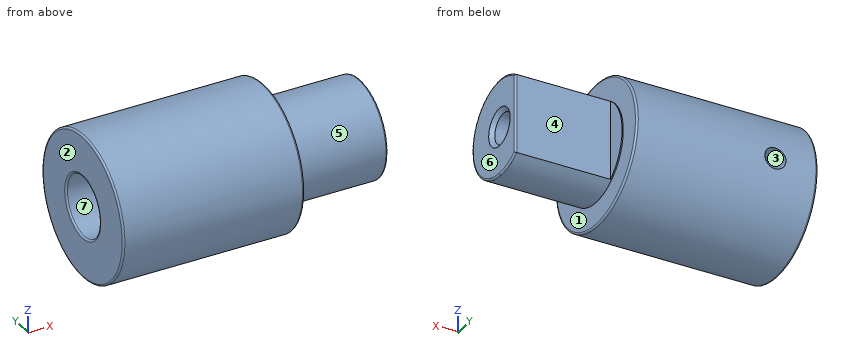
from build123d import *

# Parameters (mm, degrees)
CUT_EXTRUDE1_DEPTH          = 7.9
M3_TAPPED_HOLE1_D           = 2.5
M3_TAPPED_HOLE1_CSINK_D     = 3.15
M3_TAPPED_HOLE1_CSINK_ANGLE = 90
FILLET1_R                   = 0.15
SKETCH6_R                   = 0.875
CUT_EXTRUDE2_DEPTH          = 6


with BuildPart() as part:
    # Sketch2 → Revolve1 (revolve)
    with BuildSketch(Plane(origin=(0, 0, 0), x_dir=(1, 0, 0), z_dir=(0, 1, 0))):
        Polygon((0, 2.5), (13.1, 2.5), (13.1, 0), (23, 0), (23, 4), (15, 4), (15, 5.95), (0, 5.95), align=None)
    revolve(axis=Axis((0, 0, 0), (1, 0, 0)))

    # Sketch3 → Cut-Extrude1 (cut)
    with BuildSketch(Plane(origin=(23, 0, 0), x_dir=(0, 0, -1), z_dir=(1, 0, 0))):
        with BuildLine():
            Line((-3.272613634, 2.3), (3.272613634, 2.3))
            ThreePointArc((3.272613634, 2.3), (0, 4), (-3.272613634, 2.3))
        make_face()
    extrude(amount=-CUT_EXTRUDE1_DEPTH, mode=Mode.SUBTRACT)

    # M3 Tapped Hole1 (through all)
    with Locations(Plane(origin=(23, 0, 0), x_dir=(0, 0, 1), z_dir=(1, 0, 0))):
        with Locations((0, 0)):
            CounterSinkHole(M3_TAPPED_HOLE1_D / 2, M3_TAPPED_HOLE1_CSINK_D / 2, counter_sink_angle=M3_TAPPED_HOLE1_CSINK_ANGLE)

    # Fillet1
    fillet1_edges = [part.edges().sort_by_distance(p)[0] for p in [
        (23, -3.813820561, 1.206139599),
        (23, 2.3, 0),
        (0, 0, 2.5),
        (0, 0, 5.95),
        (15, 0, 5.95),
    ]]
    fillet(fillet1_edges, radius=FILLET1_R)

    # Sketch6 → Cut-Extrude2 (cut)
    with BuildSketch(Plane(origin=(0, 5.95, 0), x_dir=(1, 0, 0), z_dir=(0, 1, 0))):
        with Locations((3.5, 0)):
            Circle(SKETCH6_R)
    extrude(amount=-CUT_EXTRUDE2_DEPTH, mode=Mode.SUBTRACT)


solid = part.part
For this review, take the finished solid that the model builds, in its own axes (mm). Face numbers are marked on the shaded views. A direction names the side the tool comes from. Round coordinates to 2 decimals unless told otherwise and drop trailing zeros. Loops run counter-clockwise (first coordinate to the right, second up) from the corner with the lowest first, then second, coordinate; pieces in that order, holes last. Notation, with made-up numbers: (58, 2.5) - (79, 2.5) arc R16 cw to (79, 22.5) - close; hole circle Ø5 at (-35, 66.25). An arc over 180 degrees is marked (long way). Use one line per item in the form item = value.
Item 1: Mouldability with a two-part tool opening along X and no side actions: class the marked faces 1, 2, 3 and 4 as +X half, -X half, draft (parallel to the pull), parting line (faces both ways), or undercut.
Answers:
face_1 = +X half
face_2 = -X half
face_3 = undercut
face_4 = draft
Item 2: For line 1 (Y direction, x = 8.25, z = 0); line 2 (X direction, y = 4.6, z = 0) (3 decimals); line 3 (X direction, y = -2.5, z = 3.5), list the stretches that pass through material, from the lowest coordinate up.
Answers:
line_1 = -5.95 to -2.5, 2.5 to 5.95
line_2 = 0 to 2.625, 4.375 to 15
line_3 = 0 to 15
Item 3: Tool access review of the marked faces 5, 6 and 7: name each direction out of +Z, -Z, +X, -X, +Y, -Y from which nothing blocks a thin tool from reaching the whole face with its end or side.
Answers:
face_5 = +X
face_6 = +Z, -Z, +X, +Y, -Y
face_7 = -X
Item 4: Clearance check with flat-ended pins moving along their axes: P1, Ø1.1, axis at x = 3.5, z = 0, coming from the +Y side; P2, Ø4, axis at x = 20, z = 4, coming from the -Y side; P3, Ø3, axis at y = 0, z = 0, coming from the +X side (3 decimals). State where each tip first meets the part, or that it passes through.
Answers:
P1 = -2.44
P2 = -3.46
P3 = 22.925
Item 5: Consider section A-A on x = 17.25. Write out the cut boundary in (y, z), then the cut area to 3 significant figures.
Answers:
outline = (2.3, -3.27) - (2.3, 3.27) arc R4 ccw (long way) to start; hole circle Ø2.5 at (0, 0)
area = 37.6 mm^2
Item 6: Consider section B-B on x = 3.5. Write out the cut boundary in (y, z) (3 decimals), then the cut area to 3 significant figures.
Answers:
outline = (2.342, -0.875) arc R2.5 cw (long way) to (2.342, 0.875) - (5.885, 0.875) arc R5.95 ccw (long way) to (5.885, -0.875) - close
area = 85.5 mm^2
